Read the model definition and answer for the solid it produces. Units are mm, in the model's axes. A direction names the side the tool comes from. Coordinates: 2 decimals unless noted, no trailing zeros. Write each loop counter-clockwise with the first axis right and the second up, starting at its lowest first coordinate (ties: lowest second). Pieces come first, ordered by that corner, then holes.
(1) Find the intervals of material crossed by probe 1 along Z at (x, y) = (-24.5, -7.5); probe 2 along X at (y, z) = (0.5, -112); probe 3 along Y at (x, z) = (-11.5, -39.5), in increasing order.
(2) Which of the six approach directions +Z, -Z, +X, -X, +Y, -Y give full straight-line access (tool end or side, diameter ignored) to faces 1 (the flat face through (-6, -13, -120)), 2 (the cylindrical face through (29.97, 1.32, -14.93))?
(3) Section B-B on x = -25.5 is taken. Write down the section's boundary in (y, z).
(4) Section C-C on x = 0 is taken. Write down the section's boundary in (y, z).
(5) The mould has two halves that part along Z. Classify faces 3 (the flat face through (0, 0, -10)), 4 (the flat face through (0, 0, -130)), 5 (the flat face through (-6, -13, -20)): +Z half, -Z half, draft (parallel to the pull), parting line (faces both ways), or undercut.
(6) Given pin 1 (12 mm diameter, centred on x = 11, z = -38, fed in from -Y); pin 2 (12 mm diameter, centred on y = 9, z = -80, fed in from +X); pin 3 (2 mm diameter, centred on x = 3, z = -82.5, fed in from +Y); pin 4 (2 mm diameter, centred on y = 15, z = -82, fed in from +X), each flat-ended and moving along its own axis, determine where each tip first touches the part or whether it passes through.
(7) Section A-A on y = -24 is taken. Write down the section's boundary in (x, z).
from build123d import *

# Parameters (mm, degrees)
ESBO_O1_2_R             = 48.65
EXTRUSI_N_1_DEPTH       = 490
CORTE_BARRIDO_1_PITCH   = 101.6
CORTE_BARRIDO_1_HEIGHT  = 914.4
CORTE_BARRIDO_1_RADIUS  = 48.65
CROQUIS_3_RX            = 47.863125
CROQUIS_3_RY            = 47.863125
CROQUIS3_R              = 13
SALIENTE_EXTRUIR1_DEPTH = 490
CROQUIS4_R              = 49
SALIENTE_EXTRUIR2_DEPTH = 10
CROQUIS5_R              = 13.571471
SALIENTE_EXTRUIR3_DEPTH = 120
CHAFL_N2_SIZE           = 2
CROQUIS19_W             = 451.947205317
CROQUIS19_H             = 279.188572138
CORTAR_EXTRUIR4_DEPTH   = 721
CROQUIS20_R             = 30
SALIENTE_EXTRUIR4_DEPTH = 10
SALIENTE_EXTRUIR5_START = -10
CROQUIS21_R             = 30
SALIENTE_EXTRUIR5_DEPTH = 10


with BuildPart() as part:
    # Esboço1<2> → Extrusión 1 (new body)
    with BuildSketch(Plane.XY):
        Circle(ESBO_O1_2_R)
    extrude(amount=EXTRUSI_N_1_DEPTH)

    # Corte Barrido 1: sweep along a helix
    with BuildLine() as corte_barrido_1_path:
        Helix(CORTE_BARRIDO_1_PITCH, CORTE_BARRIDO_1_HEIGHT, CORTE_BARRIDO_1_RADIUS, center=(0, 0, 0), direction=(0, 0, 1), lefthand=True)
    # Croquis 3 → Corte Barrido 1 (sweep, cut)
    with BuildSketch(Plane(origin=(0, 0, 0), x_dir=(1, 0, 0), z_dir=(0, 1, 0))):
        with Locations(Location((-48.65, 0), (0, 0, -180))):
            Ellipse(CROQUIS_3_RX, CROQUIS_3_RY)
    sweep(path=corte_barrido_1_path.line, is_frenet=True, mode=Mode.SUBTRACT)

    # Croquis3 → Saliente-Extruir1 (add)
    with BuildSketch(Plane(origin=(0, 0, 0), x_dir=(-1, 0, 0), z_dir=(0, 0, -1))):
        Circle(CROQUIS3_R)
    extrude(amount=-SALIENTE_EXTRUIR1_DEPTH)

    # Croquis4 → Saliente-Extruir2 (add)
    with BuildSketch(Plane(origin=(0, 0, 0), x_dir=(-1, 0, 0), z_dir=(0, 0, -1))):
        Circle(CROQUIS4_R)
    extrude(amount=SALIENTE_EXTRUIR2_DEPTH)

    # Croquis5 → Saliente-Extruir3 (add)
    with BuildSketch(Plane(origin=(0, 0, -10), x_dir=(-1, 0, 0), z_dir=(0, 0, -1))):
        Circle(CROQUIS5_R)
    extrude(amount=SALIENTE_EXTRUIR3_DEPTH)

    # Croquis11 → Revolución1 (revolve)
    with BuildSketch(Plane(origin=(0, 0, 0), x_dir=(0, 0, -1), z_dir=(1, 0, 0)), mode=Mode.PRIVATE) as revoluci_n1_sk:
        Polygon((-490, -13), (-490, 0), (-564, 0), (-564, -6), (-526, -6), (-526, -13), (-495, -13), align=None)
    revolve(revoluci_n1_sk.sketch.rotate(Axis((0, 0, 490), (0, 0, 1)), 270), axis=Axis((0, 0, 490), (0, 0, 1)))

    # Chaflán2
    chafl_n2_edges = [part.edges().sort_by_distance(p)[0] for p in [
        (6, 0, 564),
    ]]
    chamfer(chafl_n2_edges, length=CHAFL_N2_SIZE)

    # Croquis12 → Cortar-Revolución1 (revolve, cut)
    with BuildSketch(Plane(origin=(0, 0, 0), x_dir=(1, 0, 0), z_dir=(0, 1, 0))):
        Polygon((-13, -505), (-12, -505), (-12, -509.7), (-13, -509.7), (-15.609105151, -509.7), (-15.609105151, -505), align=None)
    revolve(axis=Axis((0, 0, 526), (0, 0, -1)), mode=Mode.SUBTRACT)

    # Croquis19 → Cortar-Extruir4 (cut)
    with BuildSketch(Plane(origin=(0, 0, -10), x_dir=(-1, 0, 0), z_dir=(0, 0, -1))):
        with Locations((-30.102891015, -20.278452223)):
            Rectangle(CROQUIS19_W, CROQUIS19_H)
    extrude(amount=-CORTAR_EXTRUIR4_DEPTH, mode=Mode.SUBTRACT)

    # Croquis20 → Saliente-Extruir4 (add)
    with BuildSketch(Plane(origin=(0, 0, -10), x_dir=(-1, 0, 0), z_dir=(0, 0, -1))):
        Circle(CROQUIS20_R)
    extrude(amount=SALIENTE_EXTRUIR4_DEPTH)

    # Croquis21 → Saliente-Extruir5 (add)
    with BuildSketch(Plane(origin=(0, 0, -130), x_dir=(-1, 0, 0), z_dir=(0, 0, -1)).offset(SALIENTE_EXTRUIR5_START)):
        Circle(CROQUIS21_R)
    extrude(amount=SALIENTE_EXTRUIR5_DEPTH)


solid = part.part
Response:
1. probe 1: z = -130 to -120, -20 to -10
1. probe 2: x = -13.56 to 13.56
1. probe 3: y = -7.21 to 7.21
2. face 1: none
2. face 2: +Z, -Z
3. outline: (-15.8, -130) - (15.8, -130) - (15.8, -120) - (-15.8, -120) - close; (-15.8, -20) - (15.8, -20) - (15.8, -10) - (-15.8, -10) - close
4. outline: (-30, -130) - (30, -130) - (30, -120) - (13.57, -120) - (13.57, -20) - (30, -20) - (30, -10) - (-30, -10) - (-30, -20) - (-13.57, -20) - (-13.57, -120) - (-30, -120) - close
5. face 3: +Z half
5. face 4: -Z half
5. face 5: undercut
6. pin 1: stops at y = -12.62
6. pin 2: stops at x = 13.24
6. pin 3: stops at y = 13.42
6. pin 4: passes through
7. outline: (-18, -130) - (18, -130) - (18, -120) - (-18, -120) - close; (-18, -20) - (18, -20) - (18, -10) - (-18, -10) - close
